Can you work these out from the model? Positions are in its coordinate system, mm. Face numbers are marked on the shaded views. Round coordinates to 2 decimals unless told otherwise and drop trailing zeros. Write each loop counter-clockwise with the first axis right and the second up, starting at its lowest first coordinate (ties: lowest second). Pieces come first, ordered by that corner, then holes. Notation, with made-up numbers: M 52,5 L 69,5 A20 ccw 69,25 Z; hole C 81,81.5 d10. An arc over 180 degrees is marked long. Answer in a Markdown table with one row per item. Add a question column.
(1) If I drill on probe 1 along X at (y, z) = (25.5, 2.8); probe 2 along Y at (x, z) = (2.5, 1.95); probe 3 along X at (y, z) = (8.5, 2.3), over which ranges is the centre line in solid material (lowest first)?
(2) Suppose I cut it at A-A, the plane x = -16.5. Write out the boundary of the cut face in (y, z), then the cut area to 3 significant figures.
(3) I'm going to push a flat-ended pin straight in: pin 1 (12 mm diameter, centred on x = -38.5, y = 32.5, fed in from +Z). Where does the tip first touch, or does it pass through?
(4) Suppose I cut it at C-C, the plane x = -4. Write out the boundary of the cut face in (y, z), then the cut area to 3 significant figures.
(5) Suppose I cut it at D-D, the plane y = 40.5. Write out the boundary of the cut face in (x, z).
(6) If we mould it in two halves opening along X, with no side actions, what happens to the marked faces 1 and 2? For each: released by +X, released by -X, zero draft, split by the parting line, or undercut.
(7) Suppose I cut it at B-B, the plane y = 33.5. Write out the boundary of the cut face in (x, z).
from build123d import *

# Parameters (mm, degrees)
SKETCH_2_W          = 53.974572009
SKETCH_2_H          = 41.974503429
EXTRUDE_1_DEPTH     = 3.8
CUT_EXTRUDE_1_DEPTH = 2.3
SKETCH_4_W          = 46
SKETCH_4_H          = 34.2
CUT_EXTRUDE_2_DEPTH = 2.3
SKETCH_5_R          = 0.625
CUT_EXTRUDE_3_DEPTH = 2.8
SKETCH_7_W          = 35.12
SKETCH_7_H          = 28.19
CUT_EXTRUDE_4_DEPTH = 1.5
SKETCH_8_W          = 3
SKETCH_8_H          = 2.387251715
SKETCH_8_W_2        = 2.487286004
SKETCH_8_H_2        = 3
SKETCH_8_W_3        = 2.487286005
SKETCH_8_W_4        = 3.00002286
SKETCH_8_H_3        = 2.387274574
SKETCH_8_W_5        = 2.999984296
EXTRUDE_2_DEPTH     = 2.3
FILLET_1_R          = 1


with BuildPart() as part:
    # 草图2 → 凸台-拉伸1 (new body)
    with BuildSketch(Plane.XY):
        with Locations((-20.223936838, 24.775730738)):
            Rectangle(SKETCH_2_W, SKETCH_2_H)
    extrude(amount=EXTRUDE_1_DEPTH)

    # 草图3 → 切除-拉伸1 (cut)
    with BuildSketch(Plane.XY.offset(3.8)):
        with BuildLine():
            Line((0.763318687, 42.775657077), (0.763318687, 44.262982452))
            Line((0.763318687, 44.262982452), (-41.211192362, 44.262982452))
            Line((-41.211192362, 44.262982452), (-41.211192362, 42.775679937))
            ThreePointArc((-41.211192362, 42.775679937), (-42.093593258, 40.645375728), (-44.223897468, 39.762974832))
            Line((-44.223897468, 39.762974832), (-45.711222842, 39.762974832))
            Line((-45.711222842, 39.762974832), (-45.711222842, 9.788486643))
            Line((-45.711222842, 9.788486643), (-44.223920328, 9.788486643))
            ThreePointArc((-44.223920328, 9.788486643), (-42.093616118, 8.906085747), (-41.211215222, 6.775781538))
            Line((-41.211215222, 6.775781538), (-41.211215222, 5.288456163))
            Line((-41.211215222, 5.288456163), (0.763295827, 5.288456163))
            Line((0.763295827, 5.288456163), (0.763295827, 6.775758677))
            ThreePointArc((0.763295827, 6.775758677), (1.645696722, 8.906062887), (3.776000932, 9.788463783))
            Line((3.776000932, 9.788463783), (5.263303447, 9.788463783))
            Line((5.263303447, 9.788463783), (5.263326307, 39.762951972))
            Line((5.263326307, 39.762951972), (3.776023792, 39.762951972))
            ThreePointArc((3.776023792, 39.762951972), (1.645719582, 40.645352868), (0.763318687, 42.775657077))
        make_face()
    extrude(amount=-CUT_EXTRUDE_1_DEPTH, mode=Mode.SUBTRACT)

    # 草图4 → 切除-拉伸2 (cut)
    with BuildSketch(Plane.XY.offset(3.8)):
        with Locations((-20.223936838, 24.775730737)):
            Rectangle(SKETCH_4_W, SKETCH_4_H)
    extrude(amount=-CUT_EXTRUDE_2_DEPTH, mode=Mode.SUBTRACT)

    # 草图5 → 切除-拉伸3 (cut)
    with BuildSketch(Plane.XY.offset(3.8)):
        with Locations((-44.223897468, 42.775679937)):
            Circle(SKETCH_5_R)
        with Locations((3.776023792, 42.775679937)):
            Circle(SKETCH_5_R)
        with Locations((3.776023792, 6.775781538)):
            Circle(SKETCH_5_R)
        with Locations((-44.223897468, 6.775781538)):
            Circle(SKETCH_5_R)
    extrude(amount=-CUT_EXTRUDE_3_DEPTH, mode=Mode.SUBTRACT)

    # 草图7 → 切除-拉伸4 (cut)
    with BuildSketch(Plane(origin=(0, 0, 0), x_dir=(-1, 0, 0), z_dir=(0, 0, -1))):
        with Locations((22.913936838, 24.775730737)):
            Rectangle(SKETCH_7_W, SKETCH_7_H)
    extrude(amount=-CUT_EXTRUDE_4_DEPTH, mode=Mode.SUBTRACT)


with BuildPart() as extrude_2_tool:
    # 草图8 → 凸台-拉伸2 (new body)
    with BuildSketch(Plane.XY.offset(1.5)):
        with Locations((-39.848748169, 43.069356595)):
            Rectangle(SKETCH_8_W, SKETCH_8_H)
        with Locations((-44.46757984, 38.43376671)):
            Rectangle(SKETCH_8_W_2, SKETCH_8_H_2)
        with Locations((4.019706165, 38.43376671)):
            Rectangle(SKETCH_8_W_3, SKETCH_8_H_2)
        with Locations((-0.599125507, 43.069356595)):
            Rectangle(SKETCH_8_W, SKETCH_8_H)
        with Locations((4.019706165, 11.117694765)):
            Rectangle(SKETCH_8_W_3, SKETCH_8_H_2)
        with Locations((-44.46757984, 11.117694765)):
            Rectangle(SKETCH_8_W_2, SKETCH_8_H_2)
        with Locations((-39.848759599, 6.48209345)):
            Rectangle(SKETCH_8_W_4, SKETCH_8_H_3)
        with Locations((-0.599133359, 6.48209345)):
            Rectangle(SKETCH_8_W_5, SKETCH_8_H_3)
    extrude(amount=EXTRUDE_2_DEPTH)


with BuildPart() as part_1:
    add(part.part)


with BuildPart() as part_2:
    # 凸台-拉伸2: joined with extrude_2_tool
    add(part_1.part.fuse(extrude_2_tool.part, tol=0.00001))

    # 圆角1
    fillet_1_edges = [part_2.edges().sort_by_distance(p)[0] for p in [
        (-20.223936838, 45.762982452, 0),
        (6.763349167, 24.775730737, 0),
        (-20.223936838, 3.788479023, 0),
        (-47.211222842, 24.775730737, 0),
        (-47.211222842, 45.762982452, 1.9),
        (6.763349167, 45.762982452, 1.9),
        (6.763349167, 3.788479023, 1.9),
        (-47.211222842, 3.788479023, 1.9),
    ]]
    fillet(fillet_1_edges, radius=FILLET_1_R)


solid = part_2.part
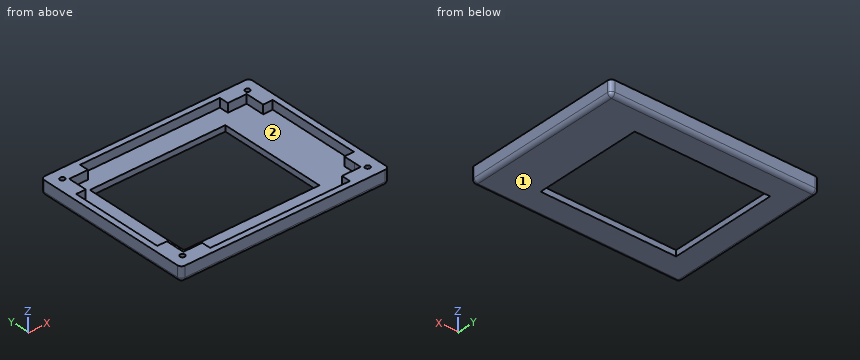
Calculated:
| question | item | result |
|---|---|---|
| 1 | probe 1 | -47.21 to -45.71, 5.26 to 6.76 |
| 1 | probe 2 | 3.79 to 7.68, 41.88 to 45.76 |
| 1 | probe 3 | -47.21 to -43.22, 2.78 to 6.76 |
| 2 | outline | M 3.79,1 A1 ccw 4.79,0 L 10.68,0 L 10.68,1.5 L 5.29,1.5 L 5.29,3.8 L 3.79,3.8 Z; M 38.87,0 L 44.76,0 A1 ccw 45.76,1 L 45.76,3.8 L 44.26,3.8 L 44.26,1.5 L 38.87,1.5 Z |
| 2 | area | 27.1 mm² |
| 3 | pin 1 | z = 1.5 |
| 4 | outline | M 3.79,1 A1 ccw 4.79,0 L 44.76,0 A1 ccw 45.76,1 L 45.76,3.8 L 44.26,3.8 L 44.26,1.5 L 5.29,1.5 L 5.29,3.8 L 3.79,3.8 Z |
| 4 | area | 69.4 mm² |
| 5 | outline | M -47.21,1 A1 ccw -46.21,0 L 5.76,0 A1 ccw 6.76,1 L 6.76,3.8 L 2.78,3.8 L 2.78,1.5 L -43.22,1.5 L -43.22,3.8 L -47.21,3.8 Z |
| 6 | face 1 | zero draft |
| 6 | face 2 | undercut |
| 7 | outline | M -47.21,1 A1 ccw -46.21,0 L -40.47,0 L -40.47,1.5 L -45.71,1.5 L -45.71,3.8 L -47.21,3.8 Z; M -5.35,0 L 5.76,0 A1 ccw 6.76,1 L 6.76,3.8 L 5.26,3.8 L 5.26,1.5 L -5.35,1.5 Z |
